Can you work these out from the model? Positions are in its coordinate system, mm. Face numbers are marked on the shaded views. A direction names the side the tool comes from. Round coordinates to 2 decimals unless told otherwise and drop trailing zeros. Order: outer loops, then holes, each group sorted by start corner. A loop starts at its lowest first (then second) coordinate and runs counter-clockwise, first axis right, second up. Notation, with made-up numbers: M 56,48.5 L 107,48.5 A11 cw 107,55.5 Z; hole C -36,73 d1. An arc over 180 degrees is marked long. Answer as a JSON object with one key per item and string values. Group by question number.
from build123d import *

# Parameters (mm, degrees)
BOSS_EXTRUDE1_DEPTH     = 7
CUT_EXTRUDE1_DEPTH      = 4
CUT_EXTRUDE1_DEPTH_BACK = 5
SKETCH2_W               = 31
SKETCH2_H               = 21


with BuildPart() as part:
    # Sketch1 → Boss-Extrude1 (new body)
    with BuildSketch(Plane(origin=(0, 0, 0), x_dir=(1, 0, 0), z_dir=(0, 1, 0))):
        with BuildLine():
            Line((-19.158798283, 16.042918455), (11.841201717, 16.042918455))
            ThreePointArc((11.841201717, 16.042918455), (15.376735623, 14.578452361), (16.841201717, 11.042918455))
            Line((16.841201717, 11.042918455), (16.841201717, -9.957081545))
            ThreePointArc((16.841201717, -9.957081545), (15.376735623, -13.492615451), (11.841201717, -14.957081545))
            Line((11.841201717, -14.957081545), (-19.158798283, -14.957081545))
            ThreePointArc((-19.158798283, -14.957081545), (-22.694332189, -13.492615451), (-24.158798283, -9.957081545))
            Line((-24.158798283, -9.957081545), (-24.158798283, 11.042918455))
            ThreePointArc((-24.158798283, 11.042918455), (-22.694332189, 14.578452361), (-19.158798283, 16.042918455))
        make_face()
    extrude(amount=BOSS_EXTRUDE1_DEPTH)

    # Sketch2 → Cut-Extrude1 (cut, two sides: drawn at the far end of the back side and taken through both)
    with BuildSketch(Plane.XZ.offset(-CUT_EXTRUDE1_DEPTH_BACK)):
        with Locations((-3.658798283, -0.542918455)):
            Rectangle(SKETCH2_W, SKETCH2_H)
    extrude(amount=CUT_EXTRUDE1_DEPTH + CUT_EXTRUDE1_DEPTH_BACK, mode=Mode.SUBTRACT)


solid = part.part
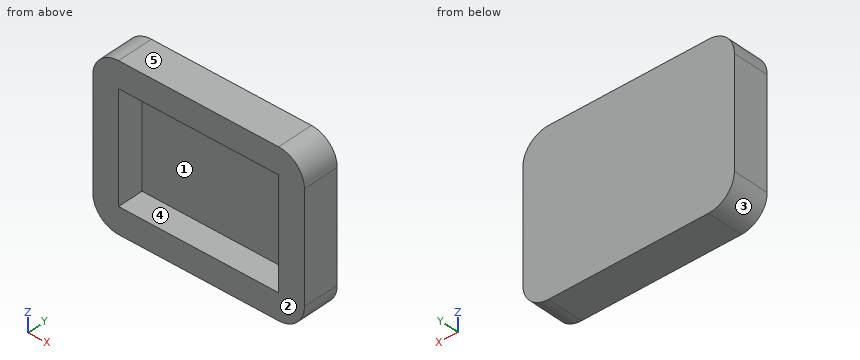
Item 1: Suppose I cut it at A-A, the plane y = 4.5. Write out the boundary of the cut face in (x, z), and give its area (3 significant figures).
Item 2: I need wall thicknesses on line 1 (Z direction, x = 1.5, y = 3.5); line 2 (X direction, y = 3, z = 1); line 3 (Y direction, x = 8.5, z = -7.5). Which ranges of each line are inside material? Lowest first, please.
Item 3: On a 3-axis mill with a long thin cutter (end or side, diameter ignored), from which of +Z, -Z, +X, -X, +Y, -Y can I reach the whole of each face in a straight line? I mean the marked faces 1 and 2. Say none if no direction works.
Item 4: Suppose I cut it at B-B, the plane z = -6.5. Write out the boundary of the cut face in (x, y).
Item 5: If we mould it in two halves opening along Z, with no side actions, what happens to the marked faces 3, 4 and 5? For each: +Z half, -Z half, draft (parallel to the pull), parting line (faces both ways), or undercut.
Item 6: Suppose I cut it at C-C, the plane x = -5. Write out the boundary of the cut face in (y, z).
Item 7: I'm going to push a flat-ended pin straight in: pin 1 Ø6.5 at (x, z) = (-10, -3) entering from -Y. Where does the tip first touch, or does it pass through?
Computed:
{
 "1": {"outline": "M -24.16,-11.04 A5 ccw -19.16,-16.04 L 11.84,-16.04 A5 ccw 16.84,-11.04 L 16.84,9.96 A5 ccw 11.84,14.96 L -19.16,14.96 A5 ccw -24.16,9.96 Z; hole M -19.16,-11.04 L 11.84,-11.04 L 11.84,9.96 L -19.16,9.96 Z", "area": "599 mm^2"},
 "2": {"line 1": "z = -16.04 to -11.04, 9.96 to 14.96", "line 2": "x = -24.16 to -19.16, 11.84 to 16.84", "line 3": "y = 5 to 7"},
 "3": {"face 1": "-Y", "face 2": "+Z, -Z, +X, -X, -Y"},
 "4": {"outline": "M -24.16,0 L -19.16,0 L -19.16,5 L 11.84,5 L 11.84,0 L 16.84,0 L 16.84,7 L -24.16,7 Z"},
 "5": {"face 3": "-Z half", "face 4": "undercut", "face 5": "+Z half"},
 "6": {"outline": "M 0,-16.04 L 7,-16.04 L 7,14.96 L 0,14.96 L 0,9.96 L 5,9.96 L 5,-11.04 L 0,-11.04 Z"},
 "7": {"pin 1": "stops at y = 5"}
}
